Geometry check sheet. Reference: drawing and pictorial views, mm from the part's lowest x, y, z. Round coordinates to 2 decimals unless told otherwise and drop trailing zeros. Order: outer loops, then holes, each group sorted by start corner. A loop starts at its lowest first (then second) coordinate and runs counter-clockwise, first axis right, second up.
(1) Sectioned sample at A-A, the plane y = 75. Enter the section's corners in (x, z).
(2) Sectioned sample at B-B, the plane z = 11. Enter the section's corners in (x, y).
(3) Sectioned sample at D-D, the plane y = 5. Enter the section's corners in (x, z).
(4) Thickness scan on probe 1 along Y at (x, z) = (6.5, 2.5); probe 2 along X at (y, z) = (60, 9.25); probe 3 along X at (y, z) = (5, 10.25). Record the ranges inside material, lowest first.
(5) Sectioned sample at C-C, the plane x = 6.35. Enter the section's corners in (y, z).
(6) Depth check by flat-ended pin: pin 1 (3 mm diameter, centred on x = 6.35, y = 20, fed in from +Z). Enter the tip coordinate at first touch or a pass-through.
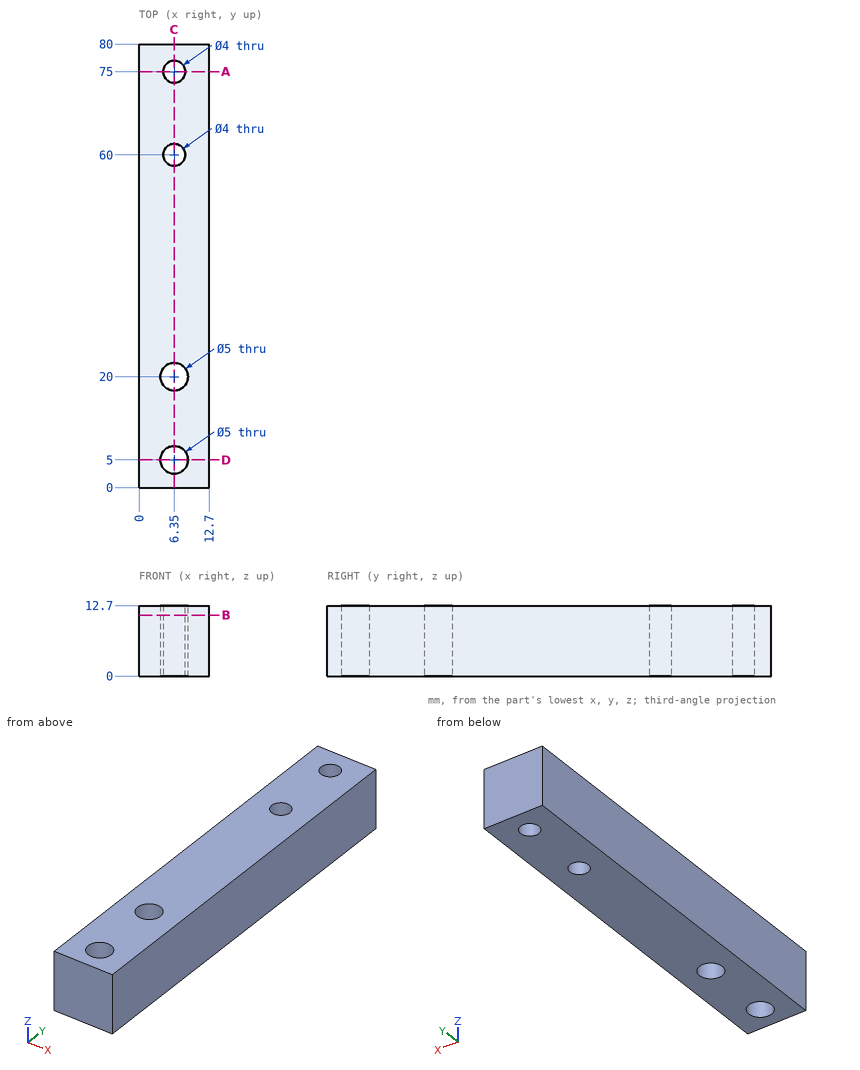
Derived:
1. outline: (0, 0) - (4.35, 0) - (4.35, 12.7) - (0, 12.7) - close; (8.35, 0) - (12.7, 0) - (12.7, 12.7) - (8.35, 12.7) - close
2. outline: (0, 0) - (12.7, 0) - (12.7, 80) - (0, 80) - close; hole circle Ø5 at (6.35, 5); hole circle Ø5 at (6.35, 20); hole circle Ø4 at (6.35, 60); hole circle Ø4 at (6.35, 75)
3. outline: (0, 0) - (3.85, 0) - (3.85, 12.7) - (0, 12.7) - close; (8.85, 0) - (12.7, 0) - (12.7, 12.7) - (8.85, 12.7) - close
4. probe 1: y = 0 to 2.5, 7.5 to 17.5, 22.5 to 58.01, 61.99 to 73.01, 76.99 to 80
4. probe 2: x = 0 to 4.35, 8.35 to 12.7
4. probe 3: x = 0 to 3.85, 8.85 to 12.7
5. outline: (0, 0) - (2.5, 0) - (2.5, 12.7) - (0, 12.7) - close; (7.5, 0) - (17.5, 0) - (17.5, 12.7) - (7.5, 12.7) - close; (22.5, 0) - (58, 0) - (58, 12.7) - (22.5, 12.7) - close; (62, 0) - (73, 0) - (73, 12.7) - (62, 12.7) - close; (77, 0) - (80, 0) - (80, 12.7) - (77, 12.7) - close
6. pin 1: passes through
